Input: part model. Units: mm. Frame: model coordinates. Face numbers are marked on the shaded views. A direction names the side the tool comes from. Round coordinates to 2 decimals unless told otherwise and drop trailing zeros. Write each loop counter-clockwise with the first axis right and the second up, starting at its lowest first coordinate (ties: lowest second). Pieces come first, ordered by that corner, then holes. Notation, with made-up numbers: M 36,88 L 40,88 A30 ccw 40,122 Z; hole C 47,2.5 d5. An arc over 180 degrees is marked long. Use one line per item in the form item = value. Start each with the question number.
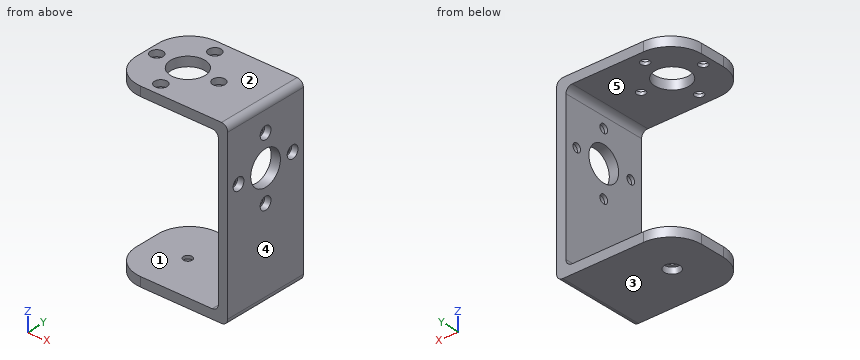
```python
from build123d import *

# Parameters (mm, degrees)
BOSS_EXTRUDE1_DEPTH = 28
SKETCH2_R           = 1.4
SKETCH2_R_2         = 5.5
CUT_EXTRUDE1_DEPTH  = 54.115440316
CUT_EXTRUDE2_REACH  = 68.287
SKETCH3_R           = 1.4
SKETCH3_R_2         = 5.5
CUT_EXTRUDE3_REACH  = 68.287
SKETCH4_R           = 1.4
SKETCH5_R           = 2
CUT_EXTRUDE4_DEPTH  = 2
SKETCH6_R           = 2
CUT_EXTRUDE5_DEPTH  = 2
SKETCH7_R           = 2.5
CUT_EXTRUDE6_DEPTH  = 2
FILLET1_R           = 10
FILLET2_R           = 2


with BuildPart() as part:
    # Sketch1 → Boss-Extrude1 (new body)
    with BuildSketch(Plane(origin=(0, 0, 0), x_dir=(1, 0, 0), z_dir=(0, 1, 0))):
        Polygon((-19, -28.5), (19, -28.5), (19, 28.5), (-19, 28.5), (-19, 25.5), (16, 25.5), (16, -25.5), (-19, -25.5), align=None)
    extrude(amount=BOSS_EXTRUDE1_DEPTH)

    # Sketch2 → Cut-Extrude1 (cut, through all)
    with BuildSketch(Plane.ZY.offset(-16)):
        with Locations((10, 4)):
            Circle(SKETCH2_R)
        with Locations((10, 24)):
            Circle(SKETCH2_R)
        with Locations((0, 14)):
            Circle(SKETCH2_R)
        with Locations((20, 14)):
            Circle(SKETCH2_R)
        with Locations((10, 14)):
            Circle(SKETCH2_R_2)
    extrude(amount=-CUT_EXTRUDE1_DEPTH, mode=Mode.SUBTRACT)

    # Sketch3 → Cut-Extrude2 (cut, up to next)
    with BuildSketch(Plane.XY.offset(28.5), mode=Mode.PRIVATE) as cut_extrude2_sk1:
        with Locations((-16, 14)):
            Circle(SKETCH3_R)
    cut_extrude2_tool1 = extrude(cut_extrude2_sk1.sketch, amount=-CUT_EXTRUDE2_REACH, mode=Mode.PRIVATE) & part.part
    # Sketch3 → Cut-Extrude2 (cut, up to next)
    with BuildSketch(Plane.XY.offset(28.5), mode=Mode.PRIVATE) as cut_extrude2_sk2:
        with Locations((-6, 4)):
            Circle(SKETCH3_R)
    cut_extrude2_tool2 = extrude(cut_extrude2_sk2.sketch, amount=-CUT_EXTRUDE2_REACH, mode=Mode.PRIVATE) & part.part
    # Sketch3 → Cut-Extrude2 (cut, up to next)
    with BuildSketch(Plane.XY.offset(28.5), mode=Mode.PRIVATE) as cut_extrude2_sk3:
        with Locations((4, 14)):
            Circle(SKETCH3_R)
    cut_extrude2_tool3 = extrude(cut_extrude2_sk3.sketch, amount=-CUT_EXTRUDE2_REACH, mode=Mode.PRIVATE) & part.part
    # Sketch3 → Cut-Extrude2 (cut, up to next)
    with BuildSketch(Plane.XY.offset(28.5), mode=Mode.PRIVATE) as cut_extrude2_sk4:
        with Locations((-6, 24)):
            Circle(SKETCH3_R)
    cut_extrude2_tool4 = extrude(cut_extrude2_sk4.sketch, amount=-CUT_EXTRUDE2_REACH, mode=Mode.PRIVATE) & part.part
    # Sketch3 → Cut-Extrude2 (cut, up to next)
    with BuildSketch(Plane.XY.offset(28.5), mode=Mode.PRIVATE) as cut_extrude2_sk5:
        with Locations((-6, 14)):
            Circle(SKETCH3_R_2)
    cut_extrude2_tool5 = extrude(cut_extrude2_sk5.sketch, amount=-CUT_EXTRUDE2_REACH, mode=Mode.PRIVATE) & part.part
    add(cut_extrude2_tool1.solids().sort_by_distance((-16, 14, 28.5))[0], mode=Mode.SUBTRACT)
    add(cut_extrude2_tool2.solids().sort_by_distance((-6, 4, 28.5))[0], mode=Mode.SUBTRACT)
    add(cut_extrude2_tool3.solids().sort_by_distance((4, 14, 28.5))[0], mode=Mode.SUBTRACT)
    add(cut_extrude2_tool4.solids().sort_by_distance((-6, 24, 28.5))[0], mode=Mode.SUBTRACT)
    add(cut_extrude2_tool5.solids().sort_by_distance((-6, 14, 28.5))[0], mode=Mode.SUBTRACT)

    # Sketch4 → Cut-Extrude3 (cut, up to next)
    with BuildSketch(Plane(origin=(0, 0, -28.5), x_dir=(-1, 0, 0), z_dir=(0, 0, -1)), mode=Mode.PRIVATE) as cut_extrude3_sk1:
        with Locations((6, 14)):
            Circle(SKETCH4_R)
    cut_extrude3_tool1 = extrude(cut_extrude3_sk1.sketch, amount=-CUT_EXTRUDE3_REACH, mode=Mode.PRIVATE) & part.part
    add(cut_extrude3_tool1.solids().sort_by_distance((-6, 14, -28.5))[0], mode=Mode.SUBTRACT)

    # Sketch5 → Cut-Extrude4 (cut)
    with BuildSketch(Plane.XY.offset(28.5)):
        with Locations((-16, 14)):
            Circle(SKETCH5_R)
        with Locations((-6, 24)):
            Circle(SKETCH5_R)
        with Locations((4, 14)):
            Circle(SKETCH5_R)
        with Locations((-6, 4)):
            Circle(SKETCH5_R)
    extrude(amount=-CUT_EXTRUDE4_DEPTH, mode=Mode.SUBTRACT)

    # Sketch6 → Cut-Extrude5 (cut)
    with BuildSketch(Plane(origin=(19, 0, 0), x_dir=(0, 0, -1), z_dir=(1, 0, 0))):
        with Locations((-10, 24)):
            Circle(SKETCH6_R)
        with Locations((0, 14)):
            Circle(SKETCH6_R)
        with Locations((-10, 4)):
            Circle(SKETCH6_R)
        with Locations((-20, 14)):
            Circle(SKETCH6_R)
    extrude(amount=-CUT_EXTRUDE5_DEPTH, mode=Mode.SUBTRACT)

    # Sketch7 → Cut-Extrude6 (cut)
    with BuildSketch(Plane(origin=(0, 0, -28.5), x_dir=(-1, 0, 0), z_dir=(0, 0, -1))):
        with Locations((6, 14)):
            Circle(SKETCH7_R)
    extrude(amount=-CUT_EXTRUDE6_DEPTH, mode=Mode.SUBTRACT)

    # Fillet1
    fillet1_edges = [part.edges().sort_by_distance(p)[0] for p in [
        (-19, 0, 27),
        (-19, 28, 27),
        (-19, 28, -27),
        (-19, 0, -27),
    ]]
    fillet(fillet1_edges, radius=FILLET1_R)

    # Fillet2
    fillet2_edges = [part.edges().sort_by_distance(p)[0] for p in [
        (19, 14, -28.5),
        (19, 14, 28.5),
        (16, 14, 25.5),
        (16, 14, -25.5),
    ]]
    fillet(fillet2_edges, radius=FILLET2_R)


solid = part.part
```
Item 1: First-contact query: pin 1 (1.7 mm diameter, centred on x = -6, y = 14, fed in from -Z); pin 2 (1.5 mm diameter, centred on x = -6, y = 13, fed in from -Z); pin 3 (2.5 mm diameter, centred on x = 4, y = 14, fed in from +Z); pin 4 (3 mm diameter, centred on x = -16, y = 14, fed in from +Z). Flat tips, straight axial feed; report the tip coordinate or a pass-through.
Item 2: Cut plane A-A (z = 20). Output: boundary loops of the cut face in (x, y).
Item 3: Draft query along Z for the marked faces 1, 2 and 3. Return one class per face: +Z half, -Z half, draft (parallel to the pull), parting line (faces both ways), or undercut.
Item 4: Cut plane C-C (x = 4). Output: boundary loops of the cut face in (y, z).
Item 5: Ray query, line 1 (Y direction, x = 18, z = 10); line 2 (Z direction, x = 9, y = 10); line 3 (Y direction, x = -6, z = 26.05). Return the intervals inside material, ascending. Write a range as from..to.
Item 6: Cut plane D-D (z = 10). Output: boundary loops of the cut face in (x, y), plus the area to 3 significant figures.
Item 7: Reachability of the marked faces 4 and 5 from +Z, -Z, +X, -X, +Y, -Y: full face, straight path, thin tool, end or side. Return the list, or none.
Item 8: Cut plane B-B (y = 4). Output: boundary loops of the cut face in (x, z), plus the area to 3 significant figures.
Final values:
q1.pin_1 = through
q1.pin_2 = -26.5
q1.pin_3 = -25.5
q1.pin_4 = 26.5
q2.outline = M 16,0 L 19,0 L 19,12 L 17,12 L 17,12.6 L 16,12.6 Z; M 16,15.4 L 17,15.4 L 17,16 L 19,16 L 19,28 L 16,28 Z
q3.face_1 = undercut
q3.face_2 = +Z half
q3.face_3 = -Z half
q4.outline = M 0,-28.5 L 28,-28.5 L 28,-25.5 L 0,-25.5 Z; M 0,25.5 L 12.6,25.5 L 12.6,26.5 L 12,26.5 L 12,28.5 L 0,28.5 Z; M 15.4,25.5 L 28,25.5 L 28,28.5 L 16,28.5 L 16,26.5 L 15.4,26.5 Z
q5.line_1 = 0..2, 6..8.5, 19.5..22, 26..28
q5.line_2 = -28.5..-25.5, 25.5..28.5
q5.line_3 = 0..2.6, 5.4..8.5, 19.5..22.6, 25.4..28
q6.outline = M 16,0 L 19,0 L 19,2 L 17,2 L 17,2.6 L 16,2.6 Z; M 16,5.4 L 17,5.4 L 17,6 L 19,6 L 19,8.5 L 16,8.5 Z; M 16,19.5 L 19,19.5 L 19,22 L 17,22 L 17,22.6 L 16,22.6 Z; M 16,25.4 L 17,25.4 L 17,26 L 19,26 L 19,28 L 16,28 Z
q6.area = 29.4 mm^2
q7.face_4 = +Z, -Z, +X, +Y, -Y
q7.face_5 = -X, +Y, -Y
q8.outline = M -17,-28.5 L 17,-28.5 A2 ccw 19,-26.5 L 19,8 L 17,8 L 17,8.6 L 16,8.6 L 16,-23.5 A2 cw 14,-25.5 L -17,-25.5 Z; M -17,25.5 L -7.4,25.5 L -7.4,26.5 L -8,26.5 L -8,28.5 L -17,28.5 Z; M -4.6,25.5 L 14,25.5 A2 cw 16,23.5 L 16,11.4 L 17,11.4 L 17,12 L 19,12 L 19,26.5 A2 ccw 17,28.5 L -4,28.5 L -4,26.5 L -4.6,26.5 Z
q8.area = 347 mm^2
